Design review of the part built by this model. Coordinates are the model's own, in mm. A direction names the side the tool comes from. Coordinates: 2 decimals unless noted, no trailing zeros. Order: outer loops, then holes, each group sorted by start corner. A loop starts at its lowest first (then second) coordinate and runs counter-clockwise, first axis right, second up. Notation, with made-up numbers: M 70.5,37.25 L 113.5,37.25 A15 cw 113.5,60.25 Z; hole C 9,-33.5 d6. An arc over 180 degrees is marked long. Use CSV: the item, a comma, the result in double quotes.
```python
from build123d import *

# Parameters (mm, degrees)
EXTRUDE_1_DEPTH     = 40
SKETCH_2_R          = 25
CUT_EXTRUDE_1_DEPTH = 20
SKETCH_3_R          = 25
CUT_EXTRUDE_2_DEPTH = 20


with BuildPart() as part:
    # 草图1 → 凸台-拉伸1 (new body)
    with BuildSketch(Plane.XY):
        with BuildLine():
            Line((0, 50), (200, 50))
            ThreePointArc((200, 50), (250, 0), (200, -50))
            Line((200, -50), (0, -50))
            ThreePointArc((0, -50), (-50, 0), (0, 50))
        make_face()
    extrude(amount=EXTRUDE_1_DEPTH)

    # 草图2 → 切除-拉伸1 (cut)
    with BuildSketch(Plane(origin=(0, 0, 0), x_dir=(-1, 0, 0), z_dir=(0, 0, -1))):
        Circle(SKETCH_2_R)
    extrude(amount=-CUT_EXTRUDE_1_DEPTH, mode=Mode.SUBTRACT)

    # 草图3 → 切除-拉伸2 (cut)
    with BuildSketch(Plane.XY.offset(40)):
        with Locations((200, 0)):
            Circle(SKETCH_3_R)
    extrude(amount=-CUT_EXTRUDE_2_DEPTH, mode=Mode.SUBTRACT)


solid = part.part
```
(1) For faces 4 (the face through (-23.846, 7.509, 9.86)), 5 (the face through (249.988, 1.099, 19.72)), 6 (the face through (200, 0, 20)), list the 3-axis set-ups (+Z, -Z, +X, -X, +Y, -Y) from which the entire face can be reached by the end or side of a thin tool; tool diameter is ignored.
The answers:
face 4,"-Z"
face 5,"+Z, -Z, +X"
face 6,"+Z"
(2) The part is to be moulded in two halves that separate along X. For faces 1 (the face through (101, -50, 20)), 2 (the face through (-49.988, -1.099, 19.72)), 3 (the face through (0, 0, 20)), say which applies: pulls with the +X half, pulls with the -X half, needs draft (parallel to the pull), parting line crosses it, or undercut.
The answers:
face 1,"needs draft"
face 2,"pulls with the -X half"
face 3,"undercut"
(3) Wall thickness on probe 1 along Y at (x, z) = (0, 12); probe 2 along Y at (x, z) = (-17.5, 14); probe 3 along Z at (x, y) = (9, -3): over which ranges is each line inside the solid? List them lowest first.
The answers:
probe 1,"y = -50 to -25, 25 to 50"
probe 2,"y = -46.84 to -17.85, 17.85 to 46.84"
probe 3,"z = 20 to 40"
(4) Add section B-B on z = 34. State the section outline as (x, y) points, and give its area (3 significant figures).
The answers:
outline,"M 0,-50 L 200,-50 A50 ccw 200,50 L 0,50 A50 ccw Z; hole C 200,0 d50"
area,"25,900 mm2"
(5) Add section C-C on x = 20. State the section outline as (y, z) points, and give its area (3 significant figures).
The answers:
outline,"M -50,0 L -15,0 L -15,20 L 15,20 L 15,0 L 50,0 L 50,40 L -50,40 Z"
area,"3,400 mm2"
(6) Add section D-D on y = 21. State the section outline as (x, z) points, and give its area (3 significant figures).
The answers:
outline,"M -45.38,0 L -13.56,0 L -13.56,20 L 13.56,20 L 13.56,0 L 245.38,0 L 245.38,40 L 213.56,40 L 213.56,20 L 186.44,20 L 186.44,40 L -45.38,40 Z"
area,"10,500 mm2"
(7) Add section A-A on y = 0. State the section outline as (x, z) points, and give its area (3 significant figures).
The answers:
outline,"M -50,0 L -25,0 L -25,20 L 25,20 L 25,0 L 250,0 L 250,40 L 225,40 L 225,20 L 175,20 L 175,40 L -50,40 Z"
area,"10,000 mm2"
(8) Clearance check with flat-ended pins moving along their axes: P1, Ø25, axis at x = -5, y = -2.5, coming from the -Z side; P2, Ø2, axis at y = 16.5, z = 21.5, coming from the -X side; P3, Ø4, axis at x = 79, y = 19.5, coming from the -Z side; P4, Ø3, axis at y = 30.5, z = 26.5, coming from the +X side. State where each tip first meets the part, or that it passes through.
The answers:
P1,"stops at z = 20"
P2,"stops at x = -47.54"
P3,"stops at z = 0"
P4,"stops at x = 240.73"
